Autodesk Inventor part; units mm, degrees
ref_plane "YZ Plane" through (0, 0, 0) normal (1, 0, 0) x (0, 1, 0)
ref_plane "XZ Plane" through (0, 0, 0) normal (0, 1, 0) x (-1, 0, 0)
ref_plane "XY Plane" through (0, 0, 0) normal (0, 0, 1) x (1, 0, 0)
sketch "Sketch1" plane through (0, 0, 0) normal (0, 1, 0) x (-1, 0, 0)
  circle A0 centre (0, 0) radius 15.875
  dimension "d0" = 31.75
extrude "Extrusion1" add sketch "Sketch1" along normal blind 12.7
sketch "Sketch4" plane through (0, 0, 0) normal (0, -1, 0) x (1, 0, 0)
  circle A0 centre (0, 0) radius 3.9688
  dimension "d18" = 7.9375
extrude "Extrusion4" add sketch "Sketch4" along normal blind 6.35
sketch "Sketch5" plane through (0, -6.35, 0) normal (0, -1, 0) x (1, 0, 0)
  line L0 (1.524, 1.524) -> (-1.524, 1.524)
  line L1 (-1.524, 1.524) -> (-1.524, -1.524)
  line L2 (-1.524, -1.524) -> (1.524, -1.524)
  line L3 (1.524, -1.524) -> (1.524, 1.524)
  line L4 (1.524, 1.524) -> (-1.524, -1.524) construction
  line L5 (-1.524, 1.524) -> (1.524, -1.524) construction
  point P0 (0, 0)
  dimension "d21" = 3.048
extrude "Extrusion5" cut sketch "Sketch5" against normal blind 19.05
properties part number "knob"
CAD build for the part. Positions are in the model's coordinates, mm. A direction names the side the tool comes from. Coordinates: 2 decimals unless noted, no trailing zeros. Write each loop counter-clockwise with the first axis right and the second up, starting at its lowest first coordinate (ties: lowest second). Pieces come first, ordered by that corner, then holes. Notation, with made-up numbers: (41.5, 24) -> (78.5, 24) arc R32 ccw to (78.5, 54) -> close; hole circle Ø5 at (77, -5.75). An arc over 180 degrees is marked (long way). Return JSON: item names as keys, results as strings. Group by question number.
Q1. Flat gauge pins, fed straight in: pin 1 (1.5 mm diameter, centred on y = -3.5, z = -1, fed in from +X); pin 2 (5 mm diameter, centred on x = 10.5, y = 9, fed in from -Z); pin 3 (4 mm diameter, centred on x = -2, y = -3, fed in from -Z). Where does each tip first touch, or does it go through?
Q2. Cut at C-C, the plane y = 4.25. Give the cut face in (x, z) (3 decimals), then the cut area to 3 significant figures.
Q3. Pull direction X, two halves, no side cores. Call faces 4 (the face through (-1.524, 3, 0)), 5 (the face through (0, -6.35, -2)), 6 (the face through (3.666, -3.131, 1.52)): released by +X, released by -X, zero draft, split by the parting line, or undercut.
Q4. Cut at D-D, the plane y = -0.5. Give the cut face in (x, z), then the cut area to 3 significant figures.
Q5. Drill centre lines: line 1 (Z direction, x = -0.5, y = 8.5); line 2 (Y direction, x = 8.5, z = -11.5); line 3 (X direction, y = -5.5, z = 1). Where is each one in solid material? Low to high.
Q6. Cut at B-B, the plane x = 0. Give the cut face in (y, z) (3 decimals), then the cut area to 3 significant figures.
Q7. Cut at A-A, the plane z = 0. Give the cut face in (x, y) (3 decimals), then the cut area to 3 significant figures.
Q8. Which spindle directions (+Z, -Z, +X, -X, +Y, -Y) get a long thin tool onto all of the face, cutting with end or side? Do faces 1 (the face through (-3, 12.7, 0)), 2 (the face through (0, 3, -1.524)), 3 (the face through (-3, 0, -3)). Say none if no direction does.
Returned:
{
 "1": {"pin 1": "stops at x = 3.96", "pin 2": "stops at z = -13.71", "pin 3": "stops at z = -3.97"},
 "2": {"outline": "circle Ø31.75 at (0, 0); hole (-1.524, -1.524) -> (1.524, -1.524) -> (1.524, 1.524) -> (-1.524, 1.524) -> close", "area": "782 mm2"},
 "3": {"face 4": "undercut", "face 5": "zero draft", "face 6": "split by the parting line"},
 "4": {"outline": "circle Ø7.94 at (0, 0); hole (-1.52, -1.52) -> (1.52, -1.52) -> (1.52, 1.52) -> (-1.52, 1.52) -> close", "area": "40.2 mm2"},
 "5": {"line 1": "z = -15.87 to -1.52, 1.52 to 15.87", "line 2": "y = 0 to 12.7", "line 3": "x = -3.84 to -1.52, 1.52 to 3.84"},
 "6": {"outline": "(-6.35, -3.969) -> (0, -3.969) -> (0, -15.875) -> (12.7, -15.875) -> (12.7, -1.524) -> (-6.35, -1.524) -> close; (-6.35, 1.524) -> (12.7, 1.524) -> (12.7, 15.875) -> (0, 15.875) -> (0, 3.969) -> (-6.35, 3.969) -> close", "area": "396 mm2"},
 "7": {"outline": "(-15.875, 0) -> (-3.969, 0) -> (-3.969, -6.35) -> (-1.524, -6.35) -> (-1.524, 12.7) -> (-15.875, 12.7) -> close; (1.524, -6.35) -> (3.969, -6.35) -> (3.969, 0) -> (15.875, 0) -> (15.875, 12.7) -> (1.524, 12.7) -> close", "area": "396 mm2"},
 "8": {"face 1": "+Z, -Z, +X, -X, +Y", "face 2": "+Y, -Y", "face 3": "-Y"}
}
